from build123d import *

# Parameters (mm, degrees)
SKETCH_1_R      = 1.65
EXTRUDE_1_DEPTH = 2


with BuildPart() as part:
    # 草图1 → 凸台-拉伸1 (new body)
    with BuildSketch(Plane.XY):
        with BuildLine():
            Line((10, 68.284271247), (10, 78.284271247))
            ThreePointArc((10, 78.284271247), (-6.350322366, 56.492864354), (0, 30))
            Line((0, 30), (0, 0))
            Line((0, 0), (10, 0))
            Line((10, 0), (10, 31.715728753))
            ThreePointArc((10, 31.715728753), (1.350167547, 50), (10, 68.284271247))
        make_face()
        with Locations((5, 5)):
            Circle(SKETCH_1_R, mode=Mode.SUBTRACT)
        with Locations((5, 17)):
            Circle(SKETCH_1_R, mode=Mode.SUBTRACT)
        with Locations((-2.697604364, 50)):
            Circle(SKETCH_1_R, mode=Mode.SUBTRACT)
        with Locations((5, 69.161348792)):
            Circle(SKETCH_1_R, mode=Mode.SUBTRACT)
        with Locations((5, 30.838651208)):
            Circle(SKETCH_1_R, mode=Mode.SUBTRACT)
    extrude(amount=EXTRUDE_1_DEPTH)


solid = part.part
The model under review builds one solid part; all positions refer to its coordinate system, in mm. A direction names the side the tool comes from. Round coordinates to 2 decimals unless told otherwise and drop trailing zeros. Loops run counter-clockwise (first coordinate to the right, second up) from the corner with the lowest first, then second, coordinate; pieces in that order, holes last. Notation, with made-up numbers: (-31.5, 89) -> (-11.5, 89) arc R30 ccw to (-11.5, 126) -> close; hole circle Ø2 at (31, -15). An arc over 180 degrees is marked (long way). Answer as CSV lines item,"result".
1) Add section A-A on y = 50. Write out the cut boundary in (x, z), plus the area to 3 significant figures.
Geometry results:
outline,"(-7.02, 0) -> (-4.35, 0) -> (-4.35, 2) -> (-7.02, 2) -> close; (-1.05, 0) -> (1.35, 0) -> (1.35, 2) -> (-1.05, 2) -> close"
area,"10.1 mm²"
2) Add section C-C on z = 0.9. Write out the cut boundary in (x, y), plus the area to 3 significant figures.
Geometry results:
outline,"(0, 0) -> (10, 0) -> (10, 31.72) arc R23.65 cw to (10, 68.28) -> (10, 78.28) arc R32.02 ccw to (0, 30) -> close; hole circle Ø3.3 at (-2.7, 50); hole circle Ø3.3 at (5, 5); hole circle Ø3.3 at (5, 17); hole circle Ø3.3 at (5, 30.84); hole circle Ø3.3 at (5, 69.16)"
area,"676 mm²"
3) Add section D-D on y = 17. Write out the cut boundary in (x, z).
Geometry results:
outline,"(0, 0) -> (3.35, 0) -> (3.35, 2) -> (0, 2) -> close; (6.65, 0) -> (10, 0) -> (10, 2) -> (6.65, 2) -> close"
4) Draft analysis for pull direction Y (two halves, no side actions). For faces 1 (the face through (4.8, 70.8, 1)), 2 (the face through (10, 73, 1)), 3 (the face through (5, 0, 1)), state which applies: pulls with the +Y half, pulls with the -Y half, needs draft (parallel to the pull), parting line crosses it, or undercut.
Geometry results:
face 1,"undercut"
face 2,"needs draft"
face 3,"pulls with the -Y half"
5) Tool access review of faces 4 (the face through (3.784, 18.115, 0.986)), 5 (the face through (0, 15, 1)): name each direction out of +Z, -Z, +X, -X, +Y, -Y from which nothing blocks a thin tool from reaching the whole face with its end or side.
Geometry results:
face 4,"+Z, -Z"
face 5,"+Z, -Z, -X, -Y"
6) Add section B-B on x = 5. Write out the cut boundary in (y, z).
Geometry results:
outline,"(0, 0) -> (3.35, 0) -> (3.35, 2) -> (0, 2) -> close; (6.65, 0) -> (15.35, 0) -> (15.35, 2) -> (6.65, 2) -> close; (18.65, 0) -> (29.19, 0) -> (29.19, 2) -> (18.65, 2) -> close; (32.49, 0) -> (37.38, 0) -> (37.38, 2) -> (32.49, 2) -> close; (62.62, 0) -> (67.51, 0) -> (67.51, 2) -> (62.62, 2) -> close; (70.81, 0) -> (75, 0) -> (75, 2) -> (70.81, 2) -> close"
7) To check wall thickness, follow line 1 along Y through (x, z) = (6, 1.4); line 2 along Y through (x, z) = (5, 1.45); line 3 along X through (y, z) = (28.5, 1.55). State the ranges of each line that lie inside material, in increasing order. Write a range as from..to.
Geometry results:
line 1,"y = 0..3.69, 6.31..15.69, 18.31..29.53, 32.15..35.92, 64.08..67.85, 70.47..75.77"
line 2,"y = 0..3.35, 6.65..15.35, 18.65..29.19, 32.49..37.38, 62.62..67.51, 70.81..75"
line 3,"x = 0..10"
